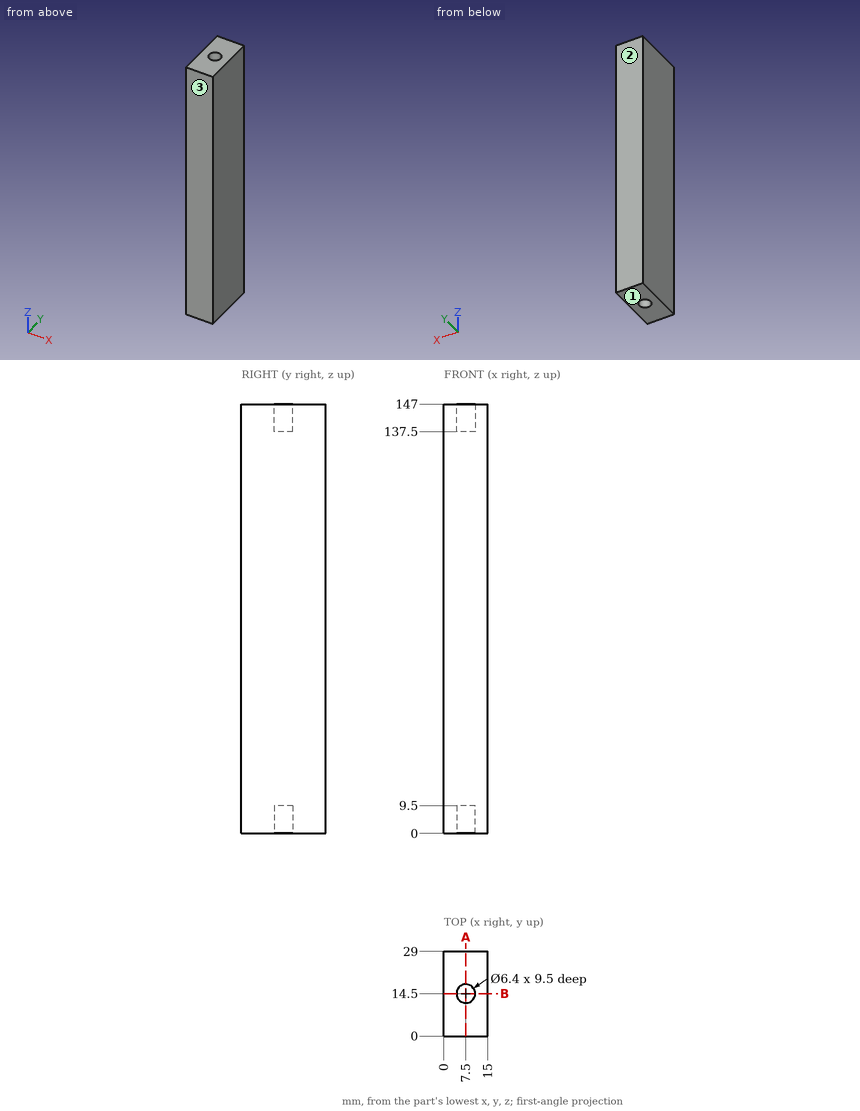
Source: three-view drawing plus pictorial views. Frame: mm from the lowest corner of the part. Round coordinates to 2 decimals unless told otherwise and drop trailing zeros. Loops run counter-clockwise (first coordinate to the right, second up) from the corner with the lowest first, then second, coordinate; pieces in that order, holes last. Notation, with made-up numbers: (2.25, -7.75) - (31.25, -7.75) arc R29 cw to (31.25, 13.25) - close; hole circle Ø7 at (88, 47). An arc over 180 degrees is marked (long way). Write each question's results on one line, items separated by ' | '. Start each with the question number.
1) First-contact query: P1, Ø6, axis at x = 7.5, y = 14.5, coming from the -Z side. Flat tip, straight axial feed; report the tip coordinate or a pass-through.
2) Cut plane A-A on x = 7.5. Return loops of the section in (y, z), then the cut area to 3 significant figures.
3) Line query: probe 1 along Y at (x, z) = (7.5, 7.25); probe 2 along Z at (x, y) = (10, 13.25). Output: solid intervals per line, ascending. Write a range as [from, to].
4) Cut plane B-B on y = 14.5. Return loops of the section in (x, z), then the cut area to 3 significant figures.
5) Mould query, pull axis Y, two halves, no side actions, for the marked faces 1, 2 and 3. Classes: released by +Y, released by -Y, zero draft, split by the parting line, or undercut.
Verdict:
1) P1: stops at z = 9.5
2) outline: (0, 0) - (11.3, 0) - (11.3, 9.5) - (17.7, 9.5) - (17.7, 0) - (29, 0) - (29, 147) - (17.7, 147) - (17.7, 137.5) - (11.3, 137.5) - (11.3, 147) - (0, 147) - close | area: 4,140 mm2
3) probe 1: y = [0, 11.3], [17.7, 29] | probe 2: z = [9.5, 137.5]
4) outline: (0, 0) - (4.3, 0) - (4.3, 9.5) - (10.7, 9.5) - (10.7, 0) - (15, 0) - (15, 147) - (10.7, 147) - (10.7, 137.5) - (4.3, 137.5) - (4.3, 147) - (0, 147) - close | area: 2,080 mm2
5) face 1: zero draft | face 2: released by +Y | face 3: released by -Y
